The figure shows three views and two pictorial views of one solid part (mm, origin at its lowest corner). Answer the questions. A direction names the side the tool comes from. Give positions to 0.01 mm unless a question says otherwise; leave off trailing zeros. Order: outer loops, then holes, each group sorted by start corner. A loop starts at its lowest first (then second) coordinate and runs counter-clockwise, first axis right, second up. Notation, with made-up numbers: (26.5, 44) - (55.5, 44) arc R18 ccw to (55.5, 77) - close; hole circle Ø5 at (-4, 51.25). An arc over 180 degrees is marked (long way). Use a Markdown table: item, result. Add a question column.
1. For a pull along X with two mould halves and no side action, classify the marked faces 4, 5, 6 and 7 as released by +X, released by -X, zero draft, split by the parting line, or undercut.
2. A cutting plane is placed at B-B on x = 33.5. Determine the outline of the cut face in (y, z), and give its area (3 significant figures).
3. A cutting plane is placed at A-A on z = 7.5. Determine the outline of the cut face in (x, y).
4. A cutting plane is placed at C-C on x = 22. Determine the outline of the cut face in (y, z).
5. Consider L1, parallel to X at y = 30.5, z = 13; L2, parallel to X at y = 22, z = 20.5; L3, parallel to Z at x = 2.5, y = 32.5. Determine where each line is inside the solid, lowest interval first.
6. A cutting plane is placed at D-D on y = 12.5. Determine the outline of the cut face in (x, z) (1 decimal).
7. Which of the six approach directions +Z, -Z, +X, -X, +Y, -Y give full straight-line access (tool end or side, diameter ignored) to the marked faces 1, 2 and 3?
8. Flat-ended cylindrical pins translate along their axes: P1, Ø5.5, axis at x = 3.5, y = 29.93, coming from the +Z side; P2, Ø4, axis at y = 33, z = 12, coming from the -X side; P3, Ø3, axis at x = 28.5, y = 30.5, coming from the +Z side. Find the tip coordinate at first contact, or state that the pin passes through.
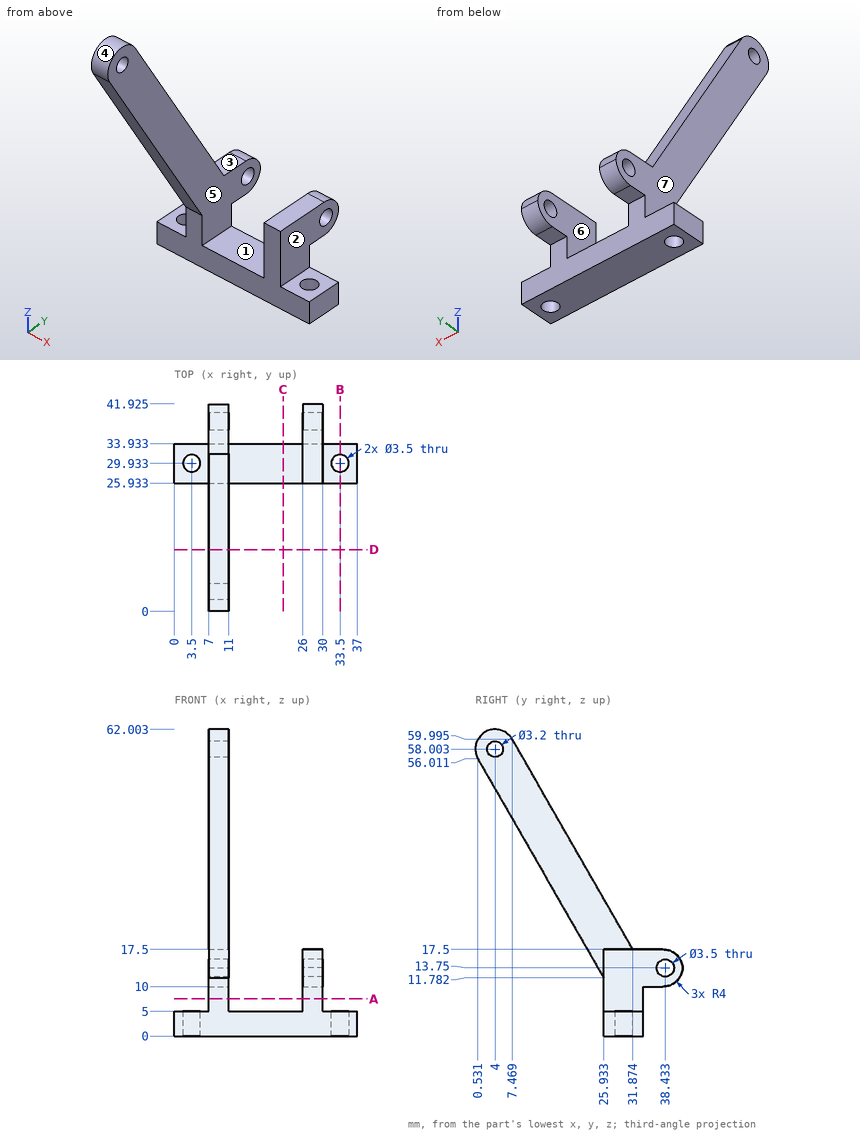
Output values:
| question | item | result |
|---|---|---|
| 1 | face 4 | zero draft |
| 1 | face 5 | undercut |
| 1 | face 6 | undercut |
| 1 | face 7 | released by -X |
| 2 | outline | (25.93, 0) - (28.18, 0) - (28.18, 5) - (25.93, 5) - close; (31.68, 0) - (33.93, 0) - (33.93, 5) - (31.68, 5) - close |
| 2 | area | 22.5 mm² |
| 3 | outline | (7, 25.93) - (11, 25.93) - (11, 33.93) - (7, 33.93) - close; (26, 25.93) - (30, 25.93) - (30, 33.93) - (26, 33.93) - close |
| 4 | outline | (25.93, 0) - (33.93, 0) - (33.93, 5) - (25.93, 5) - close |
| 5 | L1 | 7 to 11, 26 to 30 |
| 5 | L2 | 7 to 11 |
| 5 | L3 | 0 to 5 |
| 6 | outline | (7, 35.2) - (11, 35.2) - (11, 51.2) - (7, 51.2) - close |
| 7 | face 1 | +Z, +Y, -Y |
| 7 | face 2 | +Z, +X, +Y, -Y |
| 7 | face 3 | +Z, +X, -X, +Y |
| 8 | P1 | z = 5 |
| 8 | P2 | x = 7 |
| 8 | P3 | z = 17.5 |
